Here's how the part is built. I have some questions about the finished solid (model axes, mm). Face numbers are marked on the shaded views. Coordinates: 2 decimals unless noted, no trailing zeros. Loops run counter-clockwise (first coordinate to the right, second up) from the corner with the lowest first, then second, coordinate; pieces in that order, holes last.
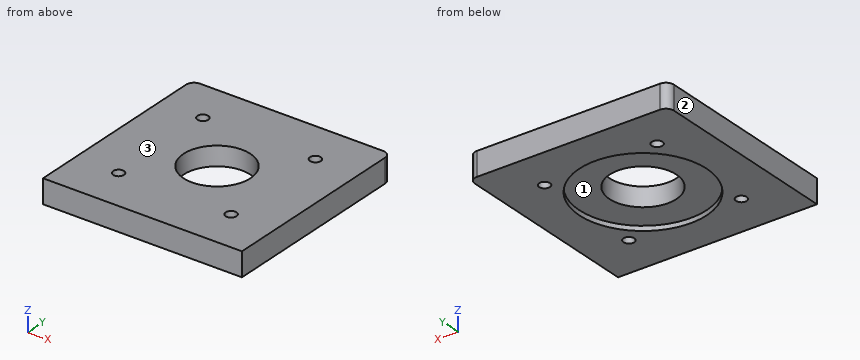
from build123d import *

# Parameters (mm, degrees)
ESQUISSE1_W             = 125
ESQUISSE1_H             = 125
BOSS_EXTRU_1_DEPTH      = 15
ESQUISSE2_R             = 40
ENL_V_MAT_EXTRU_1_DEPTH = 3
CONG_1_R                = 5
ESQUISSE11_R            = 21
ENL_V_MAT_EXTRU_2_DEPTH = 15
TROU_TARAUD_M81_D       = 6.8
TROU_TARAUD_M81_DEPTH   = 22.25
TROU_TARAUD_M81_TIP     = 2.042926105


with BuildPart() as part:
    # Esquisse1 → Boss.-Extru.1 (new body)
    with BuildSketch(Plane.XY):
        with Locations((-62.5, 62.5)):
            Rectangle(ESQUISSE1_W, ESQUISSE1_H)
    extrude(amount=BOSS_EXTRU_1_DEPTH)

    # Esquisse2 → Enlèv. mat.-Extru.1 (cut)
    with BuildSketch(Plane(origin=(0, 0, 0), x_dir=(-1, 0, 0), z_dir=(0, 0, -1))):
        with Locations((62.5, 62.5)):
            Circle(ESQUISSE2_R)
    extrude(amount=-ENL_V_MAT_EXTRU_1_DEPTH, mode=Mode.SUBTRACT)

    # Congé1
    cong_1_edges = [part.edges().sort_by_distance(p)[0] for p in [
        (-125, 125, 7.5),
        (0, 125, 7.5),
    ]]
    fillet(cong_1_edges, radius=CONG_1_R)

    # Esquisse11 → Enlèv. mat.-Extru.2 (cut)
    with BuildSketch(Plane(origin=(0, 0, 3), x_dir=(-1, 0, 0), z_dir=(0, 0, -1))):
        with Locations((62.5, 62.5)):
            Circle(ESQUISSE11_R)
    extrude(amount=-ENL_V_MAT_EXTRU_2_DEPTH, mode=Mode.SUBTRACT)

    # Trou taraudé M81
    with Locations(Plane(origin=(0, 0, 0), x_dir=(-1, 0, 0), z_dir=(0, 0, -1))):
        with Locations((97.855339059, 97.855339059), (27.144660941, 97.855339059), (27.144660941, 27.144660941), (97.855339059, 27.144660941)):
            Hole(TROU_TARAUD_M81_D / 2, depth=TROU_TARAUD_M81_DEPTH)
            with Locations((0, 0, -(TROU_TARAUD_M81_DEPTH + TROU_TARAUD_M81_TIP / 2))):  # 118° drill point
                Cone(0, TROU_TARAUD_M81_D / 2, TROU_TARAUD_M81_TIP, mode=Mode.SUBTRACT)


solid = part.part
Q1. We'd pull the mould along X, two halves only. Please class the marked faces 1, 2 and 3: pulls with the +X half, pulls with the -X half, needs draft (parallel to the pull), parting line crosses it, or undercut.
Q2. Suppose I cut it at D-D on x = -91. Write out the boundary of the cut face in (y, z).
Q3. Will these pins go through, and if not, where does the flat tip stop? P1, Ø11, axis at x = -97.86, y = 97.86, coming from the +Z side; P2, Ø24, axis at x = -79.5, y = 60, coming from the -Z side.
Q4. Please list where these lines run through material, in increasing order: probe 1 along Y at (x, z) = (-98.5, 4.25); probe 2 along Y at (x, z) = (-62.5, 9); probe 3 along Y at (x, z) = (-57.5, 13).
Q5. Suppose I cut it at A-A on y = 62.5. Write out the boundary of the cut face in (x, z), and give its area (3 significant figures).
Q6. Suppose I cut it at B-B on x = -62.5. Write out the boundary of the cut face in (y, z).
Q7. Suppose I cut it at C-C on z = 11.5. Write out the boundary of the cut face in (x, y).
Check values:
1. face 1: undercut
1. face 2: pulls with the -X half
1. face 3: needs draft
2. outline: (0, 0) - (34.43, 0) - (34.43, 3) - (90.57, 3) - (90.57, 0) - (125, 0) - (125, 15) - (0, 15) - close
3. P1: stops at z = 15
3. P2: stops at z = 3
4. probe 1: y = 0 to 23.81, 30.48 to 94.52, 101.19 to 125
4. probe 2: y = 0 to 41.5, 83.5 to 125
4. probe 3: y = 0 to 42.1, 82.9 to 125
5. outline: (-125, 0) - (-102.5, 0) - (-102.5, 3) - (-83.5, 3) - (-83.5, 15) - (-125, 15) - close; (-41.5, 3) - (-22.5, 3) - (-22.5, 0) - (0, 0) - (0, 15) - (-41.5, 15) - close
5. area: 1,130 mm2
6. outline: (0, 0) - (22.5, 0) - (22.5, 3) - (41.5, 3) - (41.5, 15) - (0, 15) - close; (83.5, 3) - (102.5, 3) - (102.5, 0) - (125, 0) - (125, 15) - (83.5, 15) - close
7. outline: (-125, 0) - (0, 0) - (0, 120) arc R5 ccw to (-5, 125) - (-120, 125) arc R5 ccw to (-125, 120) - close; hole circle Ø6.8 at (-97.86, 27.14); hole circle Ø6.8 at (-97.86, 97.86); hole circle Ø42 at (-62.5, 62.5); hole circle Ø6.8 at (-27.14, 27.14); hole circle Ø6.8 at (-27.14, 97.86)
